Could you check a few things on this model? Use its own coordinates, in mm. Face numbers are marked on the shaded views. A direction names the side the tool comes from. Give positions to 0.01 mm unless a question says otherwise; leave off trailing zeros. Loops run counter-clockwise (first coordinate to the right, second up) from the corner with the lowest first, then second, coordinate; pieces in that order, holes last. Notation, with made-up numbers: (-36.5, -35.5) - (-25.5, -35.5) arc R20 ccw to (-25.5, -1.5) - close; hole circle Ø11 at (-17, -29.75). An arc over 180 degrees is marked (long way). Write each question's results on one line, items separated by ' | '. Start each with the question number.
(1) For pin 1 (1 mm diameter, centred on x = -21.5, z = -16.5, fed in from +Y); pin 2 (7 mm diameter, centred on x = -14, y = 14, fed in from +Z); pin 3 (14 mm diameter, centred on x = -12, y = 20, fed in from -Z); pin 4 (4 mm diameter, centred on y = 3.5, z = -18.5, fed in from +X), each with a flat end and sliding along its axis, tell me the tip position at first contact or that it passes through.
(2) Suppose I cut it at A-A (x = -14). Please give me the cut outline in (y, z), and give its area (3 significant figures).
(3) Suppose I cut it at C-C (y = 14). Please give me the cut outline in (x, z).
(4) Suppose I cut it at B-B (z = -11). Please give me the cut outline in (x, y).
(5) I need wall thicknesses on line 1 (Z direction, x = -14, y = -1.2); line 2 (Y direction, x = -14, z = 1.6); line 3 (X direction, y = -1.05, z = -11). Which ranges of each line are inside material? Lowest first, please.
(6) Suppose I cut it at D-D (x = -3). Please give me the cut outline in (y, z).
(7) On a 3-axis mill with a long thin cutter (end or side, diameter ignored), from which of +Z, -Z, +X, -X, +Y, -Y can I reach the whole of each face in a straight line? I mean the marked faces 1 and 2. Say none if no direction works.
Autodesk Inventor part; units mm, degrees
ref_plane "YZ Plane" through (0, 0, 0) normal (1, 0, 0) x (0, 1, 0)
ref_plane "XZ Plane" through (0, 0, 0) normal (0, 1, 0) x (-1, 0, 0)
ref_plane "XY Plane" through (0, 0, 0) normal (0, 0, 1) x (1, 0, 0)
sketch "Sketch1" plane through (0, 0, 0) normal (0, 0, 1) x (1, 0, 0)
  line L0 (-28, 28) -> (0, 28)
  line L1 (0, 28) -> (0, 0)
  line L2 (0, 0) -> (-28, 0)
  line L3 (-28, 0) -> (-28, 28)
  dimension "d0" = 28
  dimension "d1" = 28
extrude "Extrusion1" add sketch "Sketch1" along normal blind 3
sketch "Sketch2" plane through (0, 0, 3) normal (0, 0, 1) x (1, 0, 0)
  line L0 (0, 28) -> (-28, 28)
  line L1 (0, 0) -> (0, 28)
  point P0 (-14, 14)
  dimension "d4" = 14
  dimension "d5" = 14
hole "Hole1" at (-14, 14, 3) direction (0, 0, -1) diameter 5.917 depth 19.1 tip angle 118
sketch "Sketch3" plane through (0, 0, 3) normal (0, 0, 1) x (1, 0, 0)
  line L0 (-28, 0) -> (0, 0)
  line L1 (0, 0) -> (-28, 0)
  line L2 (-28, 0) -> (-28, -3)
  line L3 (-28, -3) -> (0, -3)
  line L4 (0, -3) -> (0, 0)
  line L5 (-28, 28) -> (-28, 0)
  dimension "d13" = 3
extrude "Extrusion2" add sketch "Sketch3" against normal blind 28
sketch "Sketch4" plane through (-28, -3, 3) normal (0, -1, 0) x (1, 0, 0)
  line L0 (0, 0) -> (28, 0)
  line L1 (28, 0) -> (28, -28)
  point P0 (28, -3)
  point P1 (14, -14)
  dimension "d16" = 14
  dimension "d17" = 14
hole "Hole2" at (-14, -3, -11) direction (0, 1, 0) diameter 5.917 depth 19.1 tip angle 118
properties part number "Esquinero"
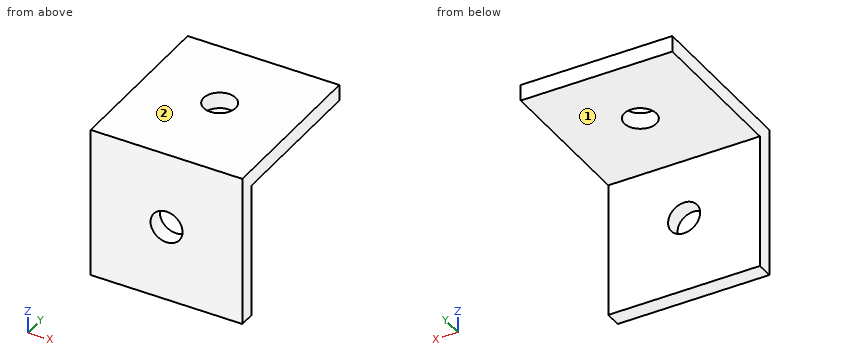
Output values:
1) pin 1: y = 0 | pin 2: z = 3 | pin 3: z = 0 | pin 4: through
2) outline: (-3, -25) - (0, -25) - (0, -13.96) - (-3, -13.96) - close; (-3, -8.04) - (0, -8.04) - (0, 0) - (11.04, 0) - (11.04, 3) - (-3, 3) - close; (16.96, 0) - (28, 0) - (28, 3) - (16.96, 3) - close | area: 132 mm2
3) outline: (-28, 0) - (-16.96, 0) - (-16.96, 3) - (-28, 3) - close; (-11.04, 0) - (0, 0) - (0, 3) - (-11.04, 3) - close
4) outline: (-28, -3) - (-16.96, -3) - (-16.96, 0) - (-28, 0) - close; (-11.04, -3) - (0, -3) - (0, 0) - (-11.04, 0) - close
5) line 1: -25 to -13.96, -8.04 to 3 | line 2: -3 to 11.04, 16.96 to 28 | line 3: -28 to -16.96, -11.04 to 0
6) outline: (-3, -25) - (0, -25) - (0, 0) - (28, 0) - (28, 3) - (-3, 3) - close
7) face 1: -Z, +X, -X, +Y | face 2: +Z, +X, -X, +Y, -Y
